The listing builds one solid part. Answer for the finished solid, in the listing's coordinates (mm). Face numbers are marked on the shaded views. A direction names the side the tool comes from. Give positions to 0.01 mm unless a question says otherwise; leave off trailing zeros. Order: outer loops, then holes, each group sorted by start corner. A loop starts at its lowest first (then second) coordinate and runs counter-clockwise, first axis right, second up. Notation, with made-up numbers: (-34, 29) - (7, 29) arc R18 ccw to (7, 37) - close; hole circle Ø4 at (86.5, 50.25). An arc over 180 degrees is marked (long way). Answer as a JSON object with one key per item and string values. Group by question number.
Q1. A cutting plane is placed at D-D, the plane y = 4.25. Give the vertices of the cut face in (x, z).
Q2. Given pin 1 (1 mm diameter, centred on y = 4, z = -1.5, fed in from +X); pin 2 (2 mm diameter, centred on x = 1.5, y = 4, fed in from -Z), each flat-ended and moving along its own axis, determine where each tip first touches the part or whether it passes through.
Q3. For the marked faces 4 and 5, determine the directions among +Z, -Z, +X, -X, +Y, -Y from which every point of the face is accessible in a straight line to the end or side of a thin tool.
Q4. Consider line 1 (Y direction, x = 2.7, z = 0); line 2 (X direction, y = 0.75, z = -1.25); line 3 (Z direction, x = 0.9, y = 3.3). Determine where each line is inside the solid, lowest interval first.
Q5. A cutting plane is placed at B-B, the plane y = 0.6. Give the vertices of the cut face in (x, z), and give its area (3 significant figures).
Q6. A cutting plane is placed at A-A, the plane z = 0. Give the vertices of the cut face in (x, y), and give its area (3 significant figures).
Q7. The mould has two halves that part along Z. Classify the marked faces 1, 2 and 3: released by +Z, released by -Z, zero draft, split by the parting line, or undercut.
Q8. A cutting plane is placed at C-C, the plane x = 2.4. Count the separate pieces of the cut face and the enclosed holes in it, and give its area (3 significant figures).
from build123d import *

# Parameters (mm, degrees)
SKETCH1_R           = 4
SKETCH1_R_2         = 3
BOSS_EXTRUDE1_DEPTH = 5
SKETCH2_W           = 1
SKETCH2_H           = 1
FILLET1_R           = 0.1


# Read off the part's stored shape, not the designer's step: Cut-Revolve-Thin1, Body-Delete/Keep 1
with BuildPart() as part:
    # Sketch1 → Boss-Extrude1 (new body)
    with BuildSketch(Plane(origin=(0, 0, 0), x_dir=(1, 0, 0), z_dir=(0, 1, 0))):
        with Locations(Location((0, 0, 0), (0, 0, 270))):
            Circle(SKETCH1_R)
        with Locations(Location((0, 0, 0), (0, 0, 270))):
            Circle(SKETCH1_R_2, mode=Mode.SUBTRACT)
    extrude(amount=BOSS_EXTRUDE1_DEPTH)

    # Sketch2 → Revolve1 (revolve)
    with BuildSketch(Plane.XY, mode=Mode.PRIVATE) as revolve1_sk:
        with Locations((-2.5, 4.5)):
            Rectangle(SKETCH2_W, SKETCH2_H)
        with Locations((-2.5, 2.5)):
            Rectangle(SKETCH2_W, SKETCH2_H)
        with Locations((-2.5, 0.5)):
            Rectangle(SKETCH2_W, SKETCH2_H)
    revolve(revolve1_sk.sketch.rotate(Axis((0, 5, 0), (0, -1, 0)), 270), axis=Axis((0, 5, 0), (0, -1, 0)))

    # Cut-Revolve-Thin1 outline → Cut-Revolve-Thin1 (revolve, cut)
    with BuildSketch(Plane.XY):
        Polygon((3.118365096, 0), (3.219907758, 0), (4, 4.424122952), (4, 5), align=None)
    revolve(axis=Axis((0, 0, 0), (0, 1, 0)), mode=Mode.SUBTRACT)

    # Body-Delete/Keep 1 outline → Body-Delete/Keep 1 (revolve, cut)
    with BuildSketch(Plane.XY):
        Polygon((4, 4.424122952), (3.219907758, 0), (4, 0), align=None)
    revolve(axis=Axis((0, 0, 0), (0, 1, 0)), mode=Mode.SUBTRACT)

    # SurfaceCut1
    split(bisect_by=Plane(origin=(0, 0, 0), x_dir=(0, 0, -1), z_dir=(1, 0, 0)), keep=Keep.TOP)

    # Fillet1
    fillet1_edges = [part.edges().sort_by_distance(p)[0] for p in [
        (2, 0, 0),
        (2, 1, 0),
        (2, 4, 0),
        (2, 5, 0),
        (2, 3, 0),
        (2, 2, 0),
    ]]
    fillet(fillet1_edges, radius=FILLET1_R)


solid = part.part
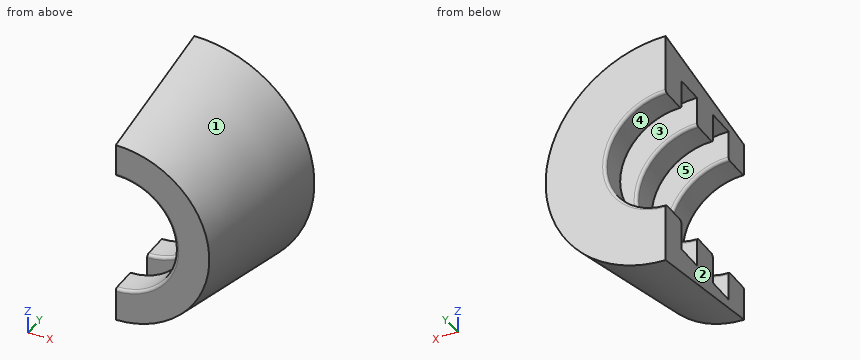
Reply:
{
 "1": {"outline": "(0, -3.87) arc R3.87 ccw to (0, 3.87) - (0, 2) arc R2 cw to (0, -2) - close"},
 "2": {"pin 1": "stops at x = 3.72", "pin 2": "stops at z = -3.87"},
 "3": {"face 4": "-X, +Y, -Y", "face 5": "-X"},
 "4": {"line 1": "y = 0 to 1, 2 to 3, 4 to 5", "line 2": "x = 1.56 to 3", "line 3": "z = -3.59 to -2.86, 2.86 to 3.59"},
 "5": {"outline": "(0, -3.22) arc R3.22 ccw to (0, 3.22) - (0, 2) arc R2 cw to (0, -2) - close", "area": "10.0 mm^2"},
 "6": {"outline": "(2, 0.1) arc R0.1 ccw to (2.1, 0) - (3.12, 0) - (4, 5) - (2.1, 5) arc R0.1 ccw to (2, 4.9) - (2, 4.1) arc R0.1 ccw to (2.1, 4) - (3, 4) - (3, 3) - (2.1, 3) arc R0.1 ccw to (2, 2.9) - (2, 2.1) arc R0.1 ccw to (2.1, 2) - (3, 2) - (3, 1) - (2.1, 1) arc R0.1 ccw to (2, 0.9) - close", "area": "5.78 mm^2"},
 "7": {"face 1": "split by the parting line", "face 2": "zero draft", "face 3": "undercut"},
 "8": {"separate pieces": "1", "enclosed holes": "2", "area": "19.0 mm^2"}
}
